Geometry check sheet. Reference: the model listing, model coordinates, mm. A direction names the side the tool comes from. Coordinates: 2 decimals unless noted, no trailing zeros. Order: outer loops, then holes, each group sorted by start corner. A loop starts at its lowest first (then second) coordinate and runs counter-clockwise, first axis right, second up.
```python
from build123d import *

# Parameters (mm, degrees)
SKETCH1_W                  = 184.15
SKETCH1_H                  = 63.5
BOSS_EXTRUDE1_DEPTH        = 9.525
SKETCH3_R                  = 14.605
CUT_EXTRUDE1_DEPTH         = 98.860072297
F_10_CLEARANCE_HOLE1_D     = 5.1054
F_6_5_6_5_DIAMETER_HOLE3_D = 6.5
SKETCH29_R                 = 15.875
CUT_EXTRUDE5_DEPTH         = 3.175
F_10_CLEARANCE_HOLE2_D     = 5.1054
SKETCH36_R                 = 2.54
CUT_EXTRUDE6_DEPTH         = 98.860072297


with BuildPart() as part:
    # Sketch1 → Boss-Extrude1 (new body)
    with BuildSketch(Plane(origin=(0, 0, 0), x_dir=(1, 0, 0), z_dir=(0, 1, 0))):
        Rectangle(SKETCH1_W, SKETCH1_H)
    extrude(amount=BOSS_EXTRUDE1_DEPTH)

    # Sketch3 → Cut-Extrude1 (cut, through all)
    with BuildSketch(Plane(origin=(0, 9.525, 0), x_dir=(1, 0, 0), z_dir=(0, 1, 0))):
        with Locations(Location((0, 0, 0), (0, 0, 270))):
            Circle(SKETCH3_R)
    extrude(amount=-CUT_EXTRUDE1_DEPTH, mode=Mode.SUBTRACT)

    # #10 Clearance Hole1 (through all)
    with Locations(Plane(origin=(0, 0, 0), x_dir=(-1, 0, 0), z_dir=(0, -1, 0))):
        with Locations((0, -25.4), (0, 25.4)):
            Hole(F_10_CLEARANCE_HOLE1_D / 2)

    # Ø6.5 (6.5) Diameter Hole3 (through all)
    with Locations(Plane(origin=(0, 0, 0), x_dir=(-1, 0, 0), z_dir=(0, -1, 0))):
        with Locations((58.039, 0), (-58.039, 0)):
            Hole(F_6_5_6_5_DIAMETER_HOLE3_D / 2)

    # Sketch29 → Cut-Extrude5 (cut)
    with BuildSketch(Plane(origin=(0, 9.525, 0), x_dir=(1, 0, 0), z_dir=(0, 1, 0))):
        with Locations(Location((0, 0, 0), (0, 0, 270))):
            Circle(SKETCH29_R)
    extrude(amount=-CUT_EXTRUDE5_DEPTH, mode=Mode.SUBTRACT)

    # #10 Clearance Hole2 (through all)
    with Locations(Plane(origin=(0, 9.525, 0), x_dir=(1, 0, 0), z_dir=(0, 1, 0))):
        with Locations((-82.55, 19.05), (-82.55, -19.05), (82.55, -19.05), (82.55, 19.05), (-82.55, 0), (82.55, 0)):
            Hole(F_10_CLEARANCE_HOLE2_D / 2)

    # Sketch36 → Cut-Extrude6 (cut, through all)
    with BuildSketch(Plane.XZ):
        with Locations(Location((-21.329210467, 13.7922, 0), (0, 0, 270))):
            Circle(SKETCH36_R)
        with Locations(Location((21.329210467, -13.7922, 0), (0, 0, 270))):
            Circle(SKETCH36_R)
    extrude(amount=-CUT_EXTRUDE6_DEPTH, mode=Mode.SUBTRACT)


solid = part.part
```
Item 1: Release check for a two-part mould opening along X. For faces 1 (the face through (-1, 0, -15)), 2 (the face through (-18.81, 4.7, 14.12)), 3 (the face through (92.075, 5, 0)) record: pulls with the +X half, pulls with the -X half, needs draft (parallel to the pull), parting line crosses it, or undercut.
Item 2: Tool access check on faces 4 (the face through (-13, 6.35, 7)), 5 (the face through (-1, 5, -31.75)). Record the directions out of +Z, -Z, +X, -X, +Y, -Y that give a thin tool (end or side, any length) a straight path to the whole face; none if there is none.
Item 3: Sectioned sample at D-D (y = 2.25). Give the number of separate pieces and of enclosed holes in the cut face, and give its area (3 significant figures).
Item 4: Sectioned sample at A-A (z = 19.05). Record the cut outline in (x, y) (3 decimals), and give its area (3 significant figures).
Item 5: Sectioned sample at B-B (x = 82.55). Record the cut outline in (y, z) (3 decimals), and give its area (3 significant figures).
Item 6: Thickness scan on line 1 along X through (y, z) = (5, 19.05) (3 decimals); line 2 along Z through (x, y) = (82.55, 2.5); line 3 along X through (y, z) = (2.25, -25) (3 decimals). Record the ranges inside material, lowest first.
Item 7: Sectioned sample at C-C (z = 0). Record the cut outline in (x, y) (3 decimals), and give its area (3 significant figures).
Geometry check:
1. face 1: needs draft
1. face 2: undercut
1. face 3: pulls with the +X half
2. face 4: +Y
2. face 5: -Z, +X, -X, +Y, -Y
3. separate pieces: 1
3. enclosed holes: 13
3. area: 10,800 mm2
4. outline: (-92.075, 0) - (-85.103, 0) - (-85.103, 9.525) - (-92.075, 9.525) - close; (-79.997, 0) - (79.997, 0) - (79.997, 9.525) - (-79.997, 9.525) - close; (85.103, 0) - (92.075, 0) - (92.075, 9.525) - (85.103, 9.525) - close
4. area: 1,660 mm2
5. outline: (0, -31.75) - (9.525, -31.75) - (9.525, -21.603) - (0, -21.603) - close; (0, -16.497) - (9.525, -16.497) - (9.525, -2.553) - (0, -2.553) - close; (0, 2.553) - (9.525, 2.553) - (9.525, 16.497) - (0, 16.497) - close; (0, 21.603) - (9.525, 21.603) - (9.525, 31.75) - (0, 31.75) - close
5. area: 459 mm2
6. line 1: x = -92.075 to -85.103, -79.997 to 79.997, 85.103 to 92.075
6. line 2: z = -31.75 to -21.6, -16.5 to -2.55, 2.55 to 16.5, 21.6 to 31.75
6. line 3: x = -92.075 to -2.521, 2.521 to 92.075
7. outline: (-92.075, 0) - (-85.103, 0) - (-85.103, 9.525) - (-92.075, 9.525) - close; (-79.997, 0) - (-61.289, 0) - (-61.289, 9.525) - (-79.997, 9.525) - close; (-54.789, 0) - (-14.605, 0) - (-14.605, 6.35) - (-15.875, 6.35) - (-15.875, 9.525) - (-54.789, 9.525) - close; (14.605, 0) - (54.789, 0) - (54.789, 9.525) - (15.875, 9.525) - (15.875, 6.35) - (14.605, 6.35) - close; (61.289, 0) - (79.997, 0) - (79.997, 9.525) - (61.289, 9.525) - close; (85.103, 0) - (92.075, 0) - (92.075, 9.525) - (85.103, 9.525) - close
7. area: 1,250 mm2
